Geometry: final body of the model. Coordinates: model frame, mm. A direction names the side the tool comes from. Give positions to 0.01 mm unless a question says otherwise; leave off trailing zeros. Order: outer loops, then holes, each group sorted by start corner. A loop starts at its lowest first (then second) coordinate and runs counter-clockwise, first axis right, second up. Notation, with made-up numbers: (62.5, 8) -> (86.5, 8) arc R13 cw to (86.5, 27) -> close; hole circle Ø4 at (79.25, 78). An arc over 180 degrees is marked (long way). Write item = value, one per line.
```python
from build123d import *

# Parameters (mm, degrees)
F0_W     = 100
F0_H     = 50
F1_DEPTH = 7.798489
F2_W     = 70
F2_H     = 20
F3_DEPTH = 20
F5_SIZE  = 2
F6_R     = 2.5
F7_DEPTH = 2


with BuildPart() as f1:
    # F0 (on Front) → F1 (new body)
    with BuildSketch(Plane.XZ):
        with Locations((50, 25)):
            Rectangle(F0_W, F0_H)
    extrude(amount=F1_DEPTH)

    # F2 (on face) → F3 (join)
    with BuildSketch(Plane.XZ.offset(7.798489)):
        with Locations((50, 25)):
            Rectangle(F2_W, F2_H)
    extrude(amount=F3_DEPTH)

    # F5
    f5_edges = [f1.edges().sort_by_distance(p)[0] for p in [
        (85, -17.798489, 15),
        (85, -17.798489, 35),
        (15, -17.798489, 15),
        (15, -17.798489, 35),
        (15, -27.798489, 25),
        (85, -27.798489, 25),
    ]]
    chamfer(f5_edges, length=F5_SIZE)

    # F6 (on face) → F7 (join)
    with BuildSketch(Plane.XZ.offset(27.798489)):
        with Locations((49.172595, 25.819309)):
            Circle(F6_R)
    extrude(amount=F7_DEPTH)


solid = f1.part
```
1) Line query: line 1 (Y direction, x = 82, z = 25); line 2 (Z direction, x = 74, y = -19); line 3 (Y direction, x = 67.5, z = 42.5). Output: solid intervals per line, ascending. Write a range as from..to.
Check sheet entries:
line_1 = -27.8..0
line_2 = 15..35
line_3 = -7.8..0
2) Section query C-C (x = 16). Output: boundary loops of the cut face in (y, z), plus the area to 3 significant figures.
Check sheet entries:
outline = (-26.8, 16) -> (-7.8, 16) -> (-7.8, 0) -> (0, 0) -> (0, 50) -> (-7.8, 50) -> (-7.8, 34) -> (-26.8, 34) -> close
area = 732 mm²
3) Reachability of faces 1 (the face through (84, -18, 34)), 2 (the face through (15, -17, 25)), 3 (the face through (16, -18, 16)), 4 (the face through (84, -18, 16)), 5 (the face through (50, -18, 35)) from +Z, -Z, +X, -X, +Y, -Y: full face, straight path, thin tool, end or side. Return the list, or none.
Check sheet entries:
face_1 = +Z, +X, -Y
face_2 = +Z, -Z, -X, -Y
face_3 = -Z, -X, -Y
face_4 = -Z, +X, -Y
face_5 = +Z, +X, -X, -Y
4) Section query D-D (z = 43). Output: boundary loops of the cut face in (x, y).
Check sheet entries:
outline = (0, -7.8) -> (100, -7.8) -> (100, 0) -> (0, 0) -> close
5) Section query B-B (x = 76). Output: boundary loops of the cut face in (y, z).
Check sheet entries:
outline = (-27.8, 15) -> (-7.8, 15) -> (-7.8, 0) -> (0, 0) -> (0, 50) -> (-7.8, 50) -> (-7.8, 35) -> (-27.8, 35) -> close
6) Section query A-A (z = 30). Output: boundary loops of the cut face in (x, y).
Check sheet entries:
outline = (0, -7.8) -> (15, -7.8) -> (15, -25.8) -> (17, -27.8) -> (83, -27.8) -> (85, -25.8) -> (85, -7.8) -> (100, -7.8) -> (100, 0) -> (0, 0) -> close
7) First-contact query: P1, Ø10, axis at x = 83.5, z = 20.5, coming from the +Y side; P2, Ø16, axis at x = 43, y = -20, coming from the -Z side; P3, Ø1.5, axis at y = -22, z = 22.5, coming from the -X side; P4, Ø6, axis at x = 46.5, y = -17, coming from the +Z side. Flat tips, straight axial feed; report the tip coordinate or a pass-through.
Check sheet entries:
P1 = 0
P2 = 15
P3 = 15
P4 = 35
